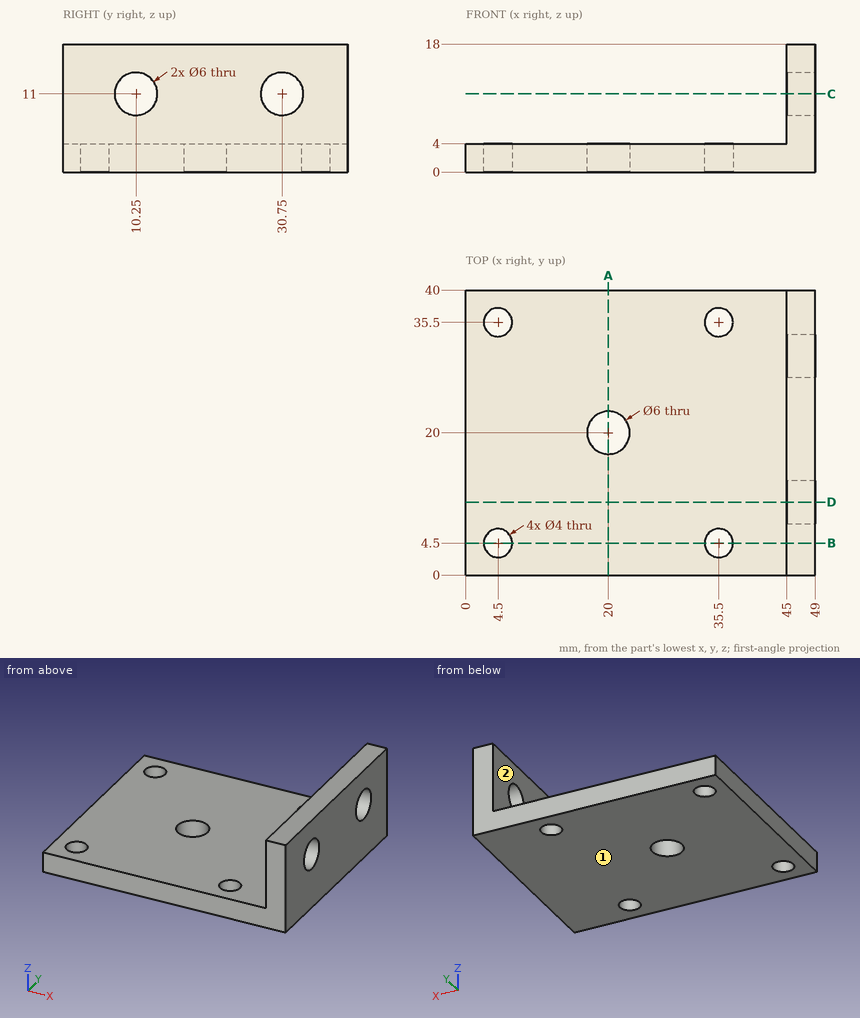
Drawing for the job (mm, zero at the part's lowest x, y, z). A direction names the side the tool comes from. Round coordinates to 2 decimals unless told otherwise and drop trailing zeros. Write each loop counter-clockwise with the first axis right and the second up, starting at its lowest first coordinate (ties: lowest second). Pieces come first, ordered by that corner, then holes. Notation, with made-up numbers: M -23,-2 L 18,-2 A27 cw 18,34 Z; hole C 58,-6 d2. An arc over 180 degrees is marked long. Answer as a JSON object with one key per item and string values. Group by question number.
(1) Cut at C-C (z = 11). Give the cut face in (x, y).
(2) Cut at D-D (y = 10.25). Give the cut face in (x, z), and give its area (3 significant figures).
(3) Cut at B-B (y = 4.5). Give the cut face in (x, z).
(4) Which spindle directions (+Z, -Z, +X, -X, +Y, -Y) get a long thin tool onto all of the face, cutting with end or side? Do the marked faces 1 and 2. Say none if no direction does.
(5) Flat gauge pins, fed straight in: pin 1 (5 mm diameter, centred on x = 15, y = 32.5, fed in from +Z); pin 2 (4 mm diameter, centred on y = 28.5, z = 8.5, fed in from -X). Where does each tip first touch, or does it go through?
(6) Drill centre lines: L1, parallel to Y at x = 4.5, z = 2.7; L2, parallel to Z at x = 16.5, y = 16; L3, parallel to Y at x = 20, z = 1.5. Where is each one in solid material? Low to high.
(7) Cut at A-A (x = 20). Give the cut face in (y, z), and give its area (3 significant figures).
Responses:
{
 "1": {"outline": "M 45,0 L 49,0 L 49,7.25 L 45,7.25 Z; M 45,13.25 L 49,13.25 L 49,27.75 L 45,27.75 Z; M 45,33.75 L 49,33.75 L 49,40 L 45,40 Z"},
 "2": {"outline": "M 0,0 L 49,0 L 49,8 L 45,8 L 45,4 L 0,4 Z; M 45,14 L 49,14 L 49,18 L 45,18 Z", "area": "228 mm2"},
 "3": {"outline": "M 0,0 L 2.5,0 L 2.5,4 L 0,4 Z; M 6.5,0 L 33.5,0 L 33.5,4 L 6.5,4 Z; M 37.5,0 L 49,0 L 49,18 L 45,18 L 45,4 L 37.5,4 Z"},
 "4": {"face 1": "-Z, +X, -X, +Y, -Y", "face 2": "+Z, -X, +Y, -Y"},
 "5": {"pin 1": "stops at z = 4", "pin 2": "stops at x = 45"},
 "6": {"L1": "y = 0 to 2.5, 6.5 to 33.5, 37.5 to 40", "L2": "z = 0 to 4", "L3": "y = 0 to 17, 23 to 40"},
 "7": {"outline": "M 0,0 L 17,0 L 17,4 L 0,4 Z; M 23,0 L 40,0 L 40,4 L 23,4 Z", "area": "136 mm2"}
}
